Check sheet for the modelled part. Datum: model origin and axes. Units: mm. A direction names the side the tool comes from. Give positions to 0.01 mm unless a question says otherwise; leave off trailing zeros. Order: outer loops, then holes, each group sorted by start corner. A loop starts at its lowest first (then second) coordinate and runs counter-clockwise, first axis right, second up. Notation, with made-up numbers: (-19, 52.25) -> (5, 52.25) arc R24 cw to (5, 63.25) -> close; hole circle Ø9 at (-14, 20). An arc over 180 degrees is marked (long way). Answer in a Markdown table with one row per item. Add a question column.
(1) Set-up check for faces 1 (the face through (0, 0, 36.83)), 2 (the face through (-2.588, -11.654, 15.027)): record each of +Z, -Z, +X, -X, +Y, -Y from which the full face is reachable in a straight line by a thin tool's end or side.
(2) Thickness scan on L1, parallel to Y at x = 4, z = 10; L2, parallel to X at y = -2, z = 13; L3, parallel to X at y = -8, z = 12.5. Record the ranges inside material, lowest first. Write a range as [from, to].
(3) Cross-section at A-A (z = 30). Record the cut outline in (x, y), then the cut area to 3 significant figures.
(4) Go/stop test with flat-tipped pins: pin 1 (5 mm diameter, centred on x = -10, z = 14.5, fed in from +Y); pin 2 (8 mm diameter, centred on x = -3, z = 10.5, fed in from -Y); pin 3 (2 mm diameter, centred on x = 1, z = 15, fed in from +Y). Record where each tip stops, or that it passes through.
```python
from build123d import *

# Parameters (mm, degrees)
F0_R     = 11.938
F1_DEPTH = 30.48
F2_R     = 16.383
F2_R_2   = 11.938
F3_DEPTH = 6.35
F4_SIZE2 = 3.5570542941
F4_SIZE  = 5.08
F5_R     = 5.08


with BuildPart() as f1:
    # F0 (on Top) → F1 (new body)
    with BuildSketch(Plane.XY):
        Circle(F0_R)
    extrude(amount=F1_DEPTH)

    # F2 (on face) → F3 (join)
    with BuildSketch(Plane.XY.offset(30.48)):
        Circle(F2_R)
        Circle(F2_R_2, mode=Mode.SUBTRACT)
        Circle(F2_R_2)
    extrude(amount=F3_DEPTH)

    # F4
    f4_edges = [f1.edges().sort_by_distance(p)[0] for p in [
        (-16.383, 0, 36.83),
    ]]
    f4_side = f1.faces().sort_by_distance((0, 0, 36.83))[0]
    chamfer(f4_edges, length=F4_SIZE, length2=F4_SIZE2, reference=f4_side)

    # F5
    f5_edges = [f1.edges().sort_by_distance(p)[0] for p in [
        (-11.303, 0, 36.83),
        (-16.383, 0, 33.272946),
    ]]
    fillet(f5_edges, radius=F5_R)


solid = f1.part
```
Answer below:
| question | item | result |
|---|---|---|
| 1 | face 1 | +Z, +X, -X, +Y, -Y |
| 1 | face 2 | -Z |
| 2 | L1 | y = [-11.25, 11.25] |
| 2 | L2 | x = [-11.77, 11.77] |
| 2 | L3 | x = [-8.86, 8.86] |
| 3 | outline | circle Ø23.88 at (0, 0) |
| 3 | area | 448 mm² |
| 4 | pin 1 | stops at y = 9.29 |
| 4 | pin 2 | stops at y = -11.94 |
| 4 | pin 3 | stops at y = 11.94 |
